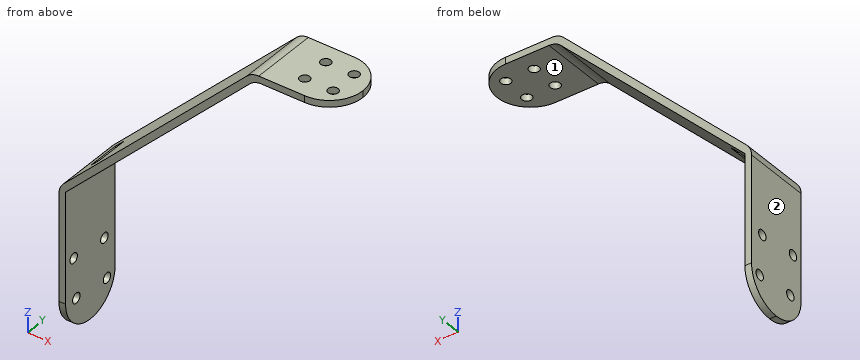
from build123d import *

# Parameters (mm, degrees)
F1_DEPTH = 20
F3_R     = 9.99999
F4_D     = 3
F5_R     = 5
F7_D     = 3
F8_W     = 4
F8_H     = 10
F9_DEPTH = 25


# Not quite as in the source:
# - a fillet or chamfer is up to 0.001 mm smaller than in the source, because OpenCascade refuses the exact size


with BuildPart() as f1:
    # F0 (on Front) → F1 (new body)
    with BuildSketch(Plane.XZ):
        Polygon((-2, 0), (0, 0), (0, 43), (56.5685424949, 99.5685424949), (81.5685424949, 99.5685424949), (81.5685424949, 101.5685424949), (55.7401153702, 101.5685424949), (-2, 43.8284271247), align=None)
    extrude(amount=F1_DEPTH)

    # F3 (radius 10 in the source; OpenCascade refuses exactly that, so slightly less here)
    f3_edges = [f1.edges().sort_by_distance(p)[0] for p in [
        (-1, -20, 0),
        (-1, 0, 0),
        (81.568542, 0, 100.568542),
        (81.568542, -20, 100.568542),
    ]]
    fillet(f3_edges, radius=F3_R)

    # F4 (through all)
    with Locations(Plane(origin=(0, 0, 99.5685424949), x_dir=(1, 0, 0), z_dir=(0, 0, -1))):
        with Locations((75.811183182, 14.2426406871), (67.3259018078, 14.2426406871), (67.3259018078, 5.7573593129), (75.811183182, 5.7573593129)):
            Hole(F4_D / 2)

    # F5
    f5_edges = [f1.edges().sort_by_distance(p)[0] for p in [
        (55.740115, -10, 101.568542),
        (56.568542, -10, 99.568542),
        (-2, -10, 43.828427),
    ]]
    fillet(f5_edges, radius=F5_R)

    # F7 (through all)
    with Locations(Plane.YZ):
        with Locations((-4.3431457505, 20.6568542495), (-16.7175144213, 21.7175144213), (-15.6568542495, 9.3431457505), (-3.2824855787, 8.2824855787)):
            Hole(F7_D / 2)

    # F8 (on face) → F9 (cut)
    with BuildSketch(Plane(origin=(-21.5, 0, 21.5), x_dir=(0.7071067812, 0, 0.7071067812), z_dir=(0.7071067812, 0, -0.7071067812))):
        with Locations((39.5918783247, 10)):
            Rectangle(F8_W, F8_H)
    extrude(amount=-F9_DEPTH, mode=Mode.SUBTRACT)


solid = f1.part
Source: CAD feature listing. Evaluate the final solid. Frame: model axes, mm. Face numbers are marked on the shaded views. A direction names the side the tool comes from. Round coordinates to 2 decimals unless told otherwise and drop trailing zeros. Loops run counter-clockwise (first coordinate to the right, second up) from the corner with the lowest first, then second, coordinate; pieces in that order, holes last.
Q1. Section A-A, the plane x = 70. Return loops of the section in (y, z).
Q2. Ray query, line 1 (Z direction, x = 67.5, y = -11); line 2 (X direction, y = -6.5, z = 35); line 3 (X direction, y = -12, z = 42.5). Return the intervals inside material, ascending.
Q3. Access query for the marked faces 1 and 2. Directions: +Z, -Z, +X, -X, +Y, -Y. A direction counts if a zero-diameter tool reaches every point of the face in a straight line with its end or side. Return the directions, or none.
Q4. First-contact query: P1, Ø6, axis at x = 51, y = -11, coming from the -Z side; P2, Ø6, axis at y = -6.5, z = 22.5, coming from the +X side; P3, Ø2, axis at y = -5, z = 45, coming from the -X side. Flat tips, straight axial feed; report the tip coordinate or a pass-through.
Q5. Section B-B, the plane z = 28.5. Return loops of the section in (x, y).
Solutions:
1. outline: (-20, 99.57) - (0, 99.57) - (0, 101.57) - (-20, 101.57) - close
2. line 1: z = 99.57 to 101.57
2. line 2: x = -2 to 0
2. line 3: x = -1.94 to 0
3. face 1: -Z, +X, +Y, -Y
3. face 2: +Z, -Z, -X, +Y, -Y
4. P1: stops at z = 91
4. P2: stops at x = 0
4. P3: stops at x = -1.47
5. outline: (-2, -20) - (0, -20) - (0, 0) - (-2, 0) - close
